```python
from build123d import *

# Parameters (mm, degrees)
SKETCH_W  = 105
SKETCH_H  = 60
SKETCH_R  = 1.63
PAD_DEPTH = 3
FILLET_R  = 3


with BuildPart() as part:
    # Sketch → Pad (new body)
    with BuildSketch(Plane.XY):
        Rectangle(SKETCH_W, SKETCH_H)
        with Locations((-46.605, -24.13)):
            Circle(SKETCH_R, mode=Mode.SUBTRACT)
        with Locations((34.67, 24.13)):
            Circle(SKETCH_R, mode=Mode.SUBTRACT)
        with BuildLine():
            ThreePointArc((-44.105, -24.13), (-44.837233, -22.362233), (-46.605, -21.63))
            ThreePointArc((-48.605, -19.63), (-48.019214, -21.044214), (-46.605, -21.63))
            Line((-48.605, 24.13), (-48.605, -19.63))
            ThreePointArc((-46.605, 26.13), (-48.019214, 25.544214), (-48.605, 24.13))
            Line((-46.605, 26.13), (30.175, 26.13))
            ThreePointArc((32.175, 24.13), (31.589213, 25.544214), (30.175, 26.13))
            ThreePointArc((32.175, 24.13), (32.905768, 22.365769), (34.67, 21.635))
            Line((34.67, 21.635), (37.07, 21.635))
            ThreePointArc((37.07, 21.635), (38.372303, 22.087576), (39.113281, 23.250234))
            ThreePointArc((45.525503, 22.5), (42.653179, 25.727981), (39.113281, 23.250234))
            ThreePointArc((45.525503, 22.5), (45.991385, 21.973349), (46.605, 21.630008))
            ThreePointArc((48.605, 19.630008), (48.019214, 21.044222), (46.605, 21.630008))
            Line((48.605, -24.129992), (48.605, 19.630008))
            ThreePointArc((46.605, -26.13), (48.019217, -25.544211), (48.605, -24.129992))
            Line((-42.105, -26.13), (46.605, -26.13))
            ThreePointArc((-44.105, -24.13), (-43.519214, -25.544214), (-42.105, -26.13))
        make_face(mode=Mode.SUBTRACT)
    extrude(amount=PAD_DEPTH)

    # Fillet
    fillet_edges = [part.edges().sort_by_distance(p)[0] for p in [
        (52.5, -30, 1.5),
        (-52.5, -30, 1.5),
        (-52.5, 30, 1.5),
        (52.5, 30, 1.5),
    ]]
    fillet(fillet_edges, radius=FILLET_R)


solid = part.part
```
Geometry: final body of the model. Coordinates: model frame, mm. A direction names the side the tool comes from. Round coordinates to 2 decimals unless told otherwise and drop trailing zeros. Loops run counter-clockwise (first coordinate to the right, second up) from the corner with the lowest first, then second, coordinate; pieces in that order, holes last.
Item 1: Section C-C, the plane x = 0.5. Output: boundary loops of the cut face in (y, z).
Checked values:
outline: (-30, 0) - (-26.13, 0) - (-26.13, 3) - (-30, 3) - close; (26.13, 0) - (30, 0) - (30, 3) - (26.13, 3) - close
Item 2: Section B-B, the plane y = -7. Output: boundary loops of the cut face in (x, z) (3 decimals).
Checked values:
outline: (-52.5, 0) - (-48.605, 0) - (-48.605, 3) - (-52.5, 3) - close; (48.605, 0) - (52.5, 0) - (52.5, 3) - (48.605, 3) - close
Item 3: Mould query, pull axis X, two halves, no side actions, for faces 1 (the flat face through (-48.605, 3, 1)), 2 (the cylindrical face through (51.6, 29.14, 1.52)), 3 (the flat face through (0, 27, 3)), 4 (the cylindrical face through (-51.64, -29.1, 1.52)). Classes: released by +X, released by -X, zero draft, split by the parting line, or undercut.
Checked values:
face 1: undercut
face 2: released by +X
face 3: zero draft
face 4: released by -X
Item 4: Line query: L1, parallel to Y at x = 34.67, z = 2 (3 decimals); L2, parallel to Y at x = -46.5, z = 1.6; L3, parallel to Y at x = -21.5, z = 1.9. Output: solid intervals per line, ascending.
Checked values:
L1: y = -30 to -26.13, 21.635 to 22.5, 25.76 to 30
L2: y = -30 to -25.76, -22.5 to -21.63, 26.13 to 30
L3: y = -30 to -26.13, 26.13 to 30
Item 5: Reachability of faces 5 (the cylindrical face through (48.004, -25.56, 1.479)), 6 (the cylindrical face through (-51.64, 29.1, 1.52)) from +Z, -Z, +X, -X, +Y, -Y: full face, straight path, thin tool, end or side. Return the list, or none.
Checked values:
face 5: +Z, -Z
face 6: +Z, -Z, -X, +Y
Item 6: Section A-A, the plane z = 1.8. State how many separate pieces and enclosed holes the cut face has, plus the area to 3 significant figures.
Checked values:
separate pieces: 1
enclosed holes: 3
area: 1,270 mm2
